Geometry: see drawing. Coordinates: mm, zero at the bounding-box minimum. Round coordinates to 2 decimals unless told otherwise and drop trailing zeros. Order: outer loops, then holes, each group sorted by start corner. A loop starts at its lowest first (then second) coordinate and runs counter-clockwise, first axis right, second up. Notation, with made-up numbers: (-34.5, 67) -> (-24.5, 67) arc R4 ccw to (-24.5, 74) -> close; hole circle Ø7 at (34.25, 59). An arc over 180 degrees is marked (long way). Answer as CSV lines item,"result". Start each with the question number.
(1) Section query A-A (x = 3.8). Output: boundary loops of the cut face in (y, z).
(2) Pull-direction query (X, two-part tool) for the marked faces 1, 2 and 3; classes: +X half, -X half, draft (parallel to the pull), parting line (faces both ways), or undercut.
(3) Section query B-B (z = 3.8). Output: boundary loops of the cut face in (x, y), plus the area to 3 significant figures.
(4) Section query C-C (y = 2.25). Output: boundary loops of the cut face in (x, z), plus the area to 3 significant figures.
(5) Line query: line 1 along X through (y, z) = (3.1, 3.75); line 2 along X through (y, z) = (3.6, 3). Output: solid intervals per line, ascending. Write a range as from..to.
(6) Contact query for a flat-ended pin moving along its axis: P1, Ø1, axis at x = 5.5, y = 2, coming from the -Z side. Output: stop coordinate, or through.
(7) Section query D-D (x = 6.5). Output: boundary loops of the cut face in (y, z).
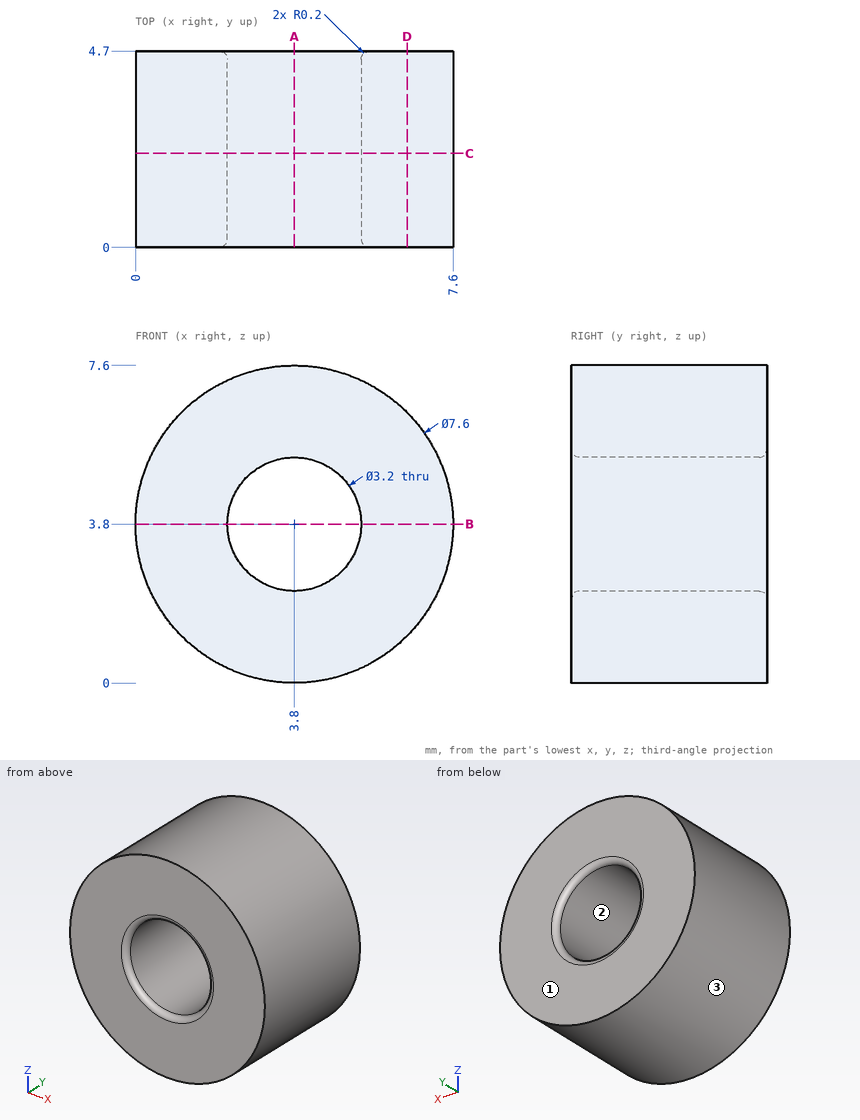
Answer block:
1,outline,"(0, 0) -> (4.7, 0) -> (4.7, 2) arc R0.2 ccw to (4.5, 2.2) -> (0.2, 2.2) arc R0.2 ccw to (0, 2) -> close; (0, 5.6) arc R0.2 ccw to (0.2, 5.4) -> (4.5, 5.4) arc R0.2 ccw to (4.7, 5.6) -> (4.7, 7.6) -> (0, 7.6) -> close"
2,face 1,"draft"
2,face 2,"undercut"
2,face 3,"parting line"
3,outline,"(0, 0) -> (2, 0) arc R0.2 ccw to (2.2, 0.2) -> (2.2, 4.5) arc R0.2 ccw to (2, 4.7) -> (0, 4.7) -> close; (5.4, 0.2) arc R0.2 ccw to (5.6, 0) -> (7.6, 0) -> (7.6, 4.7) -> (5.6, 4.7) arc R0.2 ccw to (5.4, 4.5) -> close"
3,area,"20.6 mm2"
4,outline,"circle Ø7.6 at (3.8, 3.8); hole circle Ø3.2 at (3.8, 3.8)"
4,area,"37.3 mm2"
5,line 1,"0..2.2, 5.4..7.6"
5,line 2,"0.09..2.41, 5.19..7.51"
6,P1,"z = 0.19"
7,outline,"(0, 1.13) -> (4.7, 1.13) -> (4.7, 6.47) -> (0, 6.47) -> close"
